Geometry check sheet. Reference: the model listing, model coordinates, mm. A direction names the side the tool comes from. Coordinates: 2 decimals unless noted, no trailing zeros. Write each loop counter-clockwise with the first axis right and the second up, starting at its lowest first coordinate (ties: lowest second). Pieces come first, ordered by that corner, then holes. Notation, with made-up numbers: (-2, -17) -> (42, -17) arc R16 ccw to (42, -8) -> close; hole circle Ø8 at (32.25, 64). An arc over 180 degrees is marked (long way). Answer in a Markdown table with one row per item. Add a question column.
1. Cross-section at B-B on z = -28. Record the cut outline in (x, y).
2. Set-up check for faces 1 (the cylindrical face through (-20.66, 13.17, -4.49)), 2 (the flat face through (6, -25, 30.4)), 3 (the flat face through (24, -10, -46.5)), 4 (the flat face through (-13, -21, -8.4)): record each of +Z, -Z, +X, -X, +Y, -Y from which the full face is reachable in a straight line by a thin tool's end or side.
3. Scan lines: L1, parallel to Y at x = 0, z = -25.5; L2, parallel to Y at x = 0, z = -7; L3, parallel to X at y = 23.5, z = 35. Record each from-to range of solid material in increasing order. Write a range as from..to.
4. Cross-section at A-A on z = 3.5. Record the cut outline in (x, y).
5. Mould release check, pull along Z, two halves, no side actions. Record for faces 5 (the cylindrical face through (-29.97, -1.32, 29.28)), 6 (the flat face through (0, -28, 46.5)), 7 (the flat face through (0, -28, 43.7)): pulls with the +Z half, pulls with the -Z half, needs draft (parallel to the pull), parting line crosses it, or undercut.
6. Depth check by flat-ended pin: P1, Ø4, axis at x = -22.5, z = -25, coming from the +Y side; P2, Ø6, axis at x = 16, z = 26, coming from the -Y side; P3, Ø6, axis at x = -13.5, z = 9, coming from the +Y side; P4, Ø6, axis at x = 0, y = -23.5, coming from the -Z side. Enter the tip coordinate at first touch or a pass-through.
Autodesk Inventor part; units mm, degrees
ref_plane "Arbeitsebene1" through (0, 0, 13.5) normal (0, 0, 1) x (1, 0, 0)
ref_plane "Arbeitsebene2" through (0, 0, -2.5) normal (0, 0, 1) x (1, 0, 0)
ref_plane "Arbeitsebene11" through (0, 0, 45) normal (0, 0, 1) x (1, 0, 0)
sketch "Skizze1" plane through (0, 0, 0) normal (0, 0, 1) x (1, 0, 0)
  circle A0 centre (0, 0) radius 30
  dimension "d0" = 60
extrude "Extrusion1" add sketch "Skizze1" along normal mid plane 93
ref_plane "Arbeitsebene1" through (0, 0, 13.5) normal (0, 0, 1) x (1, 0, 0)
ref_plane "Arbeitsebene2" through (0, 0, -2.5) normal (0, 0, 1) x (1, 0, 0)
ref_plane "Arbeitsebene11" through (0, 0, 45) normal (0, 0, 1) x (1, 0, 0)
sketch "Skizze12" plane through (0, 0, 13.5) normal (0, 0, 1) x (1, 0, 0)
  circle A0 centre (0, 0) radius 29.5
  circle A1 centre (0, 0) radius 30
  dimension "d91" = 0.5
extrude "Extrusion9" cut sketch "Skizze12" against normal up to surface (16 mm away)
sketch "Skizze3" plane through (0, 0, 46.5) normal (0, 0, 1) x (1, 0, 0)
  point P0 (0, 0)
  point P1 (0, 0)
hole "Bohrung1" at (0, 0, 46.5) direction (0, 0, -1) diameter 55.5 depth 15
ref_plane "Arbeitsebene13" through (0, 0, 33) normal (0, 0, 1) x (1, 0, 0)
sketch "Skizze4" plane through (0, 0, 31.5) normal (0, 0, 1) x (1, 0, 0)
  point P0 (0, 0)
  point P1 (0, 0)
hole "Bohrung2" at (0, 0, 31.5) direction (0, 0, -1) diameter 47.5 end through all
sketch "Skizze5" plane through (0, 0, -46.5) normal (0, 0, -1) x (-1, 0, 0)
  point P0 (0, 0)
  point P1 (0, 0)
hole "Bohrung3" at (0, 0, -46.5) direction (0, 0, 1) diameter 49 depth 43
sketch "Skizze6" plane through (0, 0, -46.5) normal (0, 0, -1) x (-1, 0, 0)
  circle A0 centre (0, 0) radius 27.5
  circle A1 centre (0, 0) radius 30
  dimension "d35" = 55
extrude "Extrusion3" cut sketch "Skizze6" against normal blind 12
ref_plane "Arbeitsebene4" through (0, 0, -36.5) normal (0, 0, -1) x (-1, 0, 0)
sketch "Skizze7" plane through (0, 0, -46.5) normal (0, 0, -1) x (-1, 0, 0)
  circle A0 centre (0, 0) radius 26.6
  circle A1 centre (0, 0) radius 27.5
  dimension "d39" = 53.2
ref_plane "Arbeitsebene5" through (0, 0, -34.5) normal (0, 0, -1) x (-1, 0, 0)
extrude "Extrusion4" cut sketch "Skizze7" along normal up to surface (2 mm away) from surface at -12
thread "Gewinde1"
chamfer "Fase3" distance 0.5 angle 45 1 edges at (27.5, 0, -46.5)
ref_plane "Arbeitsebene10" through (0, 0, -8.4) normal (0, 0, -1) x (-1, 0, 0)
ref_plane "Arbeitsebene9" through (0, 0, -5.5) normal (0, 0, -1) x (-1, 0, 0)
sketch "Skizze9" plane through (0, 0, -8.4) normal (0, 0, -1) x (-1, 0, 0)
  circle A0 centre (0, 0) radius 25.6
  dimension "d67" = 51.2
extrude "Extrusion6" cut sketch "Skizze9" against normal up to surface (2.9 mm away) from surface at 0
chamfer "Fase8" distance 1 angle 45 1 edges at (0, -24.5, -46.5)
ref_plane "Arbeitsebene12" through (0, 0, 33) normal (0, 0, 1) x (1, 0, 0)
sketch "Skizze10" plane through (0, 0, 31.5) normal (0, 0, 1) x (1, 0, 0)
  circle A0 centre (0, 0) radius 23.75
  circle A1 centre (0, 0) radius 25.25
  circle A2 centre (0, 0) radius 27.75
  circle A3 centre (0, 0) radius 27.75
  dimension "d76" = 1.5
  dimension "d77" = 2.5
extrude "Extrusion7" cut sketch "Skizze10" against normal blind 1.1 contours A2
ref_plane "Arbeitsebene14" through (0, 0, 41.3) normal (0, 0, 1) x (1, 0, 0)
sketch "Skizze11" plane through (0, 0, 41.3) normal (0, 0, 1) x (1, 0, 0)
  circle A0 centre (0, 0) radius 27.75
  circle A1 centre (0, 0) radius 29
  dimension "d82" = 1.25
extrude "Extrusion8" cut sketch "Skizze11" along normal blind 2.4
chamfer "Fase10" distance 1 angle 45 1 edges at (-30, 0, 46.5)
properties part number "Lampengehäuse"
Results found:
| question | item | result |
|---|---|---|
| 1 | outline | circle Ø60 at (0, 0); hole circle Ø49 at (0, 0) |
| 2 | face 1 | -Z |
| 2 | face 2 | +Z |
| 2 | face 3 | -Z, +X, -X, +Y, -Y |
| 2 | face 4 | none |
| 3 | L1 | y = -30..-24.5, 24.5..30 |
| 3 | L2 | y = -30..-25.6, 25.6..30 |
| 3 | L3 | x = -18.65..-14.76, 14.76..18.65 |
| 4 | outline | circle Ø59 at (0, 0); hole circle Ø47.5 at (0, 0) |
| 5 | face 5 | needs draft |
| 5 | face 6 | pulls with the +Z half |
| 5 | face 7 | undercut |
| 6 | P1 | stops at y = 21.9 |
| 6 | P2 | stops at y = -27.04 |
| 6 | P3 | stops at y = 27.57 |
| 6 | P4 | stops at z = -46.5 |
